Part model, mm, in its own coordinate system. Face numbers are marked on the shaded views. A direction names the side the tool comes from. Round coordinates to 2 decimals unless told otherwise and drop trailing zeros. Order: outer loops, then holes, each group sorted by start corner. A loop starts at its lowest first (then second) coordinate and runs counter-clockwise, first axis right, second up. Notation, with made-up numbers: (10.5, -18.5) - (34.5, -18.5) arc R19 cw to (34.5, -2.5) - close; hole circle Ø10 at (46.5, 66). An arc over 180 degrees is marked (long way). Return JSON: item names as keys, results as strings. Group by question number.
Item 1: Two-plate mould, pull along X, no slides. Class the marked faces 1, 2, 3 and 4: released by +X, released by -X, zero draft, split by the parting line, or undercut.
Item 2: Saw through at B-B on x = 9.5. List the corners of the cut face in (y, z), and give its area (3 significant figures).
Item 3: Saw through at C-C on z = 0.75. List the corners of the cut face in (x, y), and give its area (3 significant figures).
Item 4: Probe probe 1 along X at (y, z) = (-11.5, -1.75); probe 2 along Y at (x, z) = (0, -4); probe 3 along Y at (x, z) = (-9.89, 0.75). List the from-to ranges inside material, lowest first.
Item 5: Saw through at A-A on y = -12. State how many separate pieces and enclosed holes the cut face has, and give its area (3 significant figures).
Item 6: Tool access for the marked faces 5, 6, 7 and 8: list every direction of +Z, -Z, +X, -X, +Y, -Y with a clear straight run to the whole face (end or side of a thin tool).
Item 7: Drop flat-ended pins along their axis: pin 1 (4.5 mm diameter, centred on y = 4, z = -1.5, fed in from +X); pin 2 (0.5 mm diameter, centred on x = 0, z = 3, fed in from +Y) (3 decimals); pin 3 (0.5 mm diameter, centred on y = -7, z = 1, fed in from +X). Give the stop position or say it passes through.
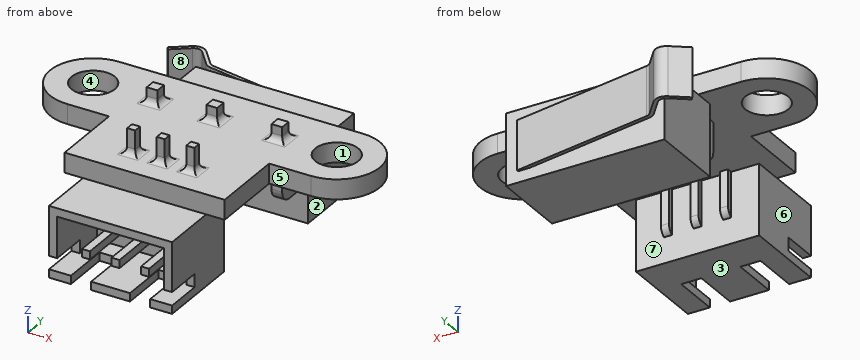
```python
from build123d import *

# Parameters (mm, degrees)
SKETCH1_R           = 1.75
BOSS_EXTRUDE1_DEPTH = 1.6
SKETCH2_W           = 12.85
SKETCH2_H           = 6.2
BOSS_EXTRUDE2_DEPTH = 5.8
BOSS_EXTRUDE3_DEPTH = 2
SKETCH4_W           = 0.87
SKETCH4_H           = 0.87
SKETCH6_W           = 10
SKETCH6_H           = 7
BOSS_EXTRUDE4_DEPTH = 5.73
SKETCH7_W           = 8.66
SKETCH7_H           = 4.39
CUT_EXTRUDE1_DEPTH  = 5.35
SKETCH8_W           = 1.64
SKETCH8_H           = 0.67
CUT_EXTRUDE2_DEPTH  = 3.86
SKETCH9_W           = 0.67
SKETCH9_H           = 1.07
CUT_EXTRUDE3_DEPTH  = 3.04
SKETCH11_W          = 0.65
SKETCH11_H          = 0.65
FILLET1_R           = 0.508


with BuildPart() as part:
    # Sketch1 → Boss-Extrude1 (new body)
    with BuildSketch(Plane.XY):
        with BuildLine():
            Line((-9.890000015, 3.499999985), (9.890000015, 3.499999985))
            ThreePointArc((9.890000015, 3.499999985), (13.39, 0), (9.890000015, -3.499999985))
            Line((9.890000015, -3.499999985), (6.5, -3.499999985))
            Line((6.5, -3.499999985), (6.5, -9.500000015))
            Line((6.5, -9.500000015), (-6.5, -9.500000015))
            Line((-6.5, -9.500000015), (-6.5, -3.499999985))
            Line((-6.5, -3.499999985), (-9.890000015, -3.499999985))
            ThreePointArc((-9.890000015, -3.499999985), (-13.39, 0), (-9.890000015, 3.499999985))
        make_face()
        with Locations((-9.890000015, 0)):
            Circle(SKETCH1_R, mode=Mode.SUBTRACT)
        with Locations((9.890000015, 0)):
            Circle(SKETCH1_R, mode=Mode.SUBTRACT)
    extrude(amount=BOSS_EXTRUDE1_DEPTH)

    # Sketch2 → Boss-Extrude2 (add)
    with BuildSketch(Plane(origin=(0, 0, 0), x_dir=(-1, 0, 0), z_dir=(0, 0, -1))):
        with Locations((0, 4.979999985)):
            Rectangle(SKETCH2_W, SKETCH2_H)
    extrude(amount=BOSS_EXTRUDE2_DEPTH)

    # Sketch3 → Boss-Extrude3 (add, symmetric)
    with BuildSketch(Plane.XY.offset(-2.9)):
        with BuildLine():
            Line((5.449691358, 8.227953818), (-6.259057602, 10.18197492))
            ThreePointArc((-6.259057602, 10.18197492), (-6.460661712, 10.25352545), (-6.625323786, 10.390090807))
            Line((-6.625323786, 10.390090807), (-7.732620651, 11.697470228))
            ThreePointArc((-7.732620651, 11.697470228), (-8.324478366, 12.014086654), (-8.972711282, 11.839915469))
            Line((-8.972711282, 11.839915469), (-10.347606141, 10.817657467))
            Line((-10.347606141, 10.817657467), (-10.168606555, 10.576910404))
            Line((-10.168606555, 10.576910404), (-8.793711695, 11.599168407))
            ThreePointArc((-8.793711695, 11.599168407), (-8.358713291, 11.716046438), (-7.961545614, 11.503580153))
            Line((-7.961545614, 11.503580153), (-6.854248749, 10.196200732))
            ThreePointArc((-6.854248749, 10.196200732), (-6.608869972, 9.992691572), (-6.308440318, 9.886067253))
            Line((-6.308440318, 9.886067253), (5.400308642, 7.932046152))
            Line((5.400308642, 7.932046152), (5.449691358, 8.227953818))
        make_face()
    extrude(amount=BOSS_EXTRUDE3_DEPTH, both=True)

    # Sweep3: sweep along a path in Sketch5
    with BuildLine(Plane(origin=(0, 0, 0), x_dir=(0, 0, -1), z_dir=(1, 0, 0))) as sweep3_path:
        Line((2.9, 1.879999985), (2.9, 0.508))
        ThreePointArc((2.9, 0.508), (2.751210245, 0.148789755), (2.392, 0))
        Line((2.392, 0), (-2.8, 0))
    # Sketch4 → Sweep3 (sweep)
    with BuildSketch(Plane.XZ.offset(-1.879999985)):
        with Locations((-4.8475, -2.9)):
            Rectangle(SKETCH4_W, SKETCH4_H)
        with Locations((0, -2.9)):
            Rectangle(SKETCH4_W, SKETCH4_H)
        with Locations((5.2825, -2.9)):
            Rectangle(SKETCH4_W, SKETCH4_H)
    sweep(path=sweep3_path.line)

    # Sketch6 → Boss-Extrude4 (add)
    with BuildSketch(Plane(origin=(0, 0, 0), x_dir=(-1, 0, 0), z_dir=(0, 0, -1))):
        with Locations((0, -10.600000015)):
            Rectangle(SKETCH6_W, SKETCH6_H)
    extrude(amount=BOSS_EXTRUDE4_DEPTH)

    # Sketch7 → Cut-Extrude1 (cut)
    with BuildSketch(Plane.XZ.offset(14.100000015)):
        with Locations((0, -2.865)):
            Rectangle(SKETCH7_W, SKETCH7_H)
    extrude(amount=-CUT_EXTRUDE1_DEPTH, mode=Mode.SUBTRACT)

    # Sketch8 → Cut-Extrude2 (cut)
    with BuildSketch(Plane(origin=(0, -14.100000015, 0), x_dir=(-1, 0, 0), z_dir=(0, -1, 0))):
        with Locations((2.4, 5.395)):
            Rectangle(SKETCH8_W, SKETCH8_H)
        with Locations((-2.4, 5.395)):
            Rectangle(SKETCH8_W, SKETCH8_H)
    extrude(amount=-CUT_EXTRUDE2_DEPTH, mode=Mode.SUBTRACT)

    # Sketch9 → Cut-Extrude3 (cut)
    with BuildSketch(Plane.XZ.offset(14.100000015)):
        with Locations((-4.665, -4.525)):
            Rectangle(SKETCH9_W, SKETCH9_H)
        with Locations((4.665, -4.525)):
            Rectangle(SKETCH9_W, SKETCH9_H)
    extrude(amount=-CUT_EXTRUDE3_DEPTH, mode=Mode.SUBTRACT)

    # Sweep4: sweep along a path in Sketch10
    with BuildLine(Plane(origin=(0, 0, 0), x_dir=(0, 0, -1), z_dir=(1, 0, 0))) as sweep4_path:
        Line((3.43, -13.430000015), (3.43, -7.508000015))
        ThreePointArc((3.43, -7.508000015), (3.281210245, -7.14878977), (2.922, -7.000000015))
        Line((2.922, -7.000000015), (-3.6, -7.000000015))
    # Sketch11 → Sweep4 (sweep)
    with BuildSketch(Plane(origin=(0, -13.430000015, 0), x_dir=(1, 0, 0), z_dir=(0, 1, 0))):
        with Locations((-2.4, 3.43)):
            Rectangle(SKETCH11_W, SKETCH11_H)
        with Locations((0, 3.43)):
            Rectangle(SKETCH11_W, SKETCH11_H)
        with Locations((2.4, 3.43)):
            Rectangle(SKETCH11_W, SKETCH11_H)
    sweep(path=sweep4_path.line)

    # Fillet1
    fillet1_edges = [part.edges().sort_by_distance(p)[0] for p in [
        (0, 0.435, 1.6),
        (0.435, 0, 1.6),
        (0, -0.435, 1.6),
        (-0.435, 0, 1.6),
        (5.2825, 0.435, 1.6),
        (5.7175, 0, 1.6),
        (5.2825, -0.435, 1.6),
        (4.8475, 0, 1.6),
        (-2.4, -6.675000015, 1.6),
        (-2.4, -7.325000015, 1.6),
        (-2.725, -7.000000015, 1.6),
        (-2.075, -7.000000015, 1.6),
        (0, -6.675000015, 1.6),
        (0, -7.325000015, 1.6),
        (-0.325, -7.000000015, 1.6),
        (0.325, -7.000000015, 1.6),
        (2.4, -6.675000015, 1.6),
        (2.4, -7.325000015, 1.6),
        (2.075, -7.000000015, 1.6),
        (2.725, -7.000000015, 1.6),
        (-4.8475, 0.435, 1.6),
        (-4.4125, 0, 1.6),
        (-4.8475, -0.435, 1.6),
        (-5.2825, 0, 1.6),
    ]]
    fillet(fillet1_edges, radius=FILLET1_R)


solid = part.part
```
Filled in:
{
 "1": {"face 1": "undercut", "face 2": "released by +X", "face 3": "zero draft", "face 4": "undercut"},
 "2": {"outline": "(-3.5, 0) - (-1.71, 0) - (-1.71, 1.6) - (-3.5, 1.6) - close; (1.71, 0) - (3.5, 0) - (3.5, 1.6) - (1.71, 1.6) - close", "area": "5.74 mm^2"},
 "3": {"outline": "(-9.89, -3.5) - (-6.5, -3.5) - (-6.5, -9.5) - (6.5, -9.5) - (6.5, -3.5) - (9.89, -3.5) arc R3.5 ccw to (9.89, 3.5) - (-9.89, 3.5) arc R3.5 ccw to start; hole circle Ø3.5 at (-9.89, 0); hole circle Ø3.5 at (9.89, 0)", "area": "236 mm^2"},
 "4": {"probe 1": "x = -5 to -4.33, 4.33 to 5", "probe 2": "y = -8.75 to -7.1, 1.88 to 8.08, 8.83 to 9.14", "probe 3": "y = -3.5 to -1.75, 1.75 to 3.5"},
 "5": {"separate pieces": "7", "enclosed holes": "0", "area": "16.9 mm^2"},
 "6": {"face 5": "+Z, -Z, +X, -Y", "face 6": "-Z, -X, -Y", "face 7": "-Z", "face 8": "+Z, -Z, -Y"},
 "7": {"pin 1": "stops at x = 12.51", "pin 2": "stops at y = 0.435", "pin 3": "stops at x = 6.5"}
}
